```python
from build123d import *

# Parameters (mm, degrees)
SKETCH1_W              = 25.4
SKETCH1_H              = 25.4
SKETCH1_W_2            = 19.05
SKETCH1_H_2            = 19.05
BOSS_EXTRUDE1_DEPTH    = 347.345
F_10_CLEARANCE_HOLE1_D = 5.1054
F_10_CLEARANCE_HOLE2_D = 5.1054


with BuildPart() as part:
    # Sketch1 → Boss-Extrude1 (new body)
    with BuildSketch(Plane(origin=(0, 0, 0), x_dir=(1, 0, 0), z_dir=(0, 1, 0))):
        Rectangle(SKETCH1_W, SKETCH1_H)
        Rectangle(SKETCH1_W_2, SKETCH1_H_2, mode=Mode.SUBTRACT)
    extrude(amount=BOSS_EXTRUDE1_DEPTH)

    # #10 Clearance Hole1 (through all)
    with Locations(Plane.XY.offset(12.7)):
        with Locations((0, 283.845), (0, 12.7), (0, 38.1), (0, 63.5), (0, 334.645), (0, 309.245)):
            Hole(F_10_CLEARANCE_HOLE1_D / 2)

    # #10 Clearance Hole2 (through all)
    with Locations(Plane(origin=(-1665.705302189, -475.547296868, 15.875), x_dir=(1, 0, 0), z_dir=(0, 0, 1))):
        with Locations((1665.705300516, 564.447296868), (1665.705300516, 733.992296868)):
            Hole(F_10_CLEARANCE_HOLE2_D / 2)


solid = part.part
```
Check sheet for the modelled part. Datum: model origin and axes. Units: mm. A direction names the side the tool comes from. Coordinates: 2 decimals unless noted, no trailing zeros. Loops run counter-clockwise (first coordinate to the right, second up) from the corner with the lowest first, then second, coordinate; pieces in that order, holes last.
1) Access from +Z, -Z, +X, -X, +Y, -Y to the whole of each face (thin tool, end or side, straight path). Record for faces 1 (the face through (0, 171, 9.525)), 2 (the face through (0, 171, 12.7)).
2) Release check for a two-part mould opening along X. For faces 3 (the face through (-12.7, 171, 0)), 4 (the face through (9.525, 171, 0)), 5 (the face through (0, 171, -12.7)), 6 (the face through (12.7, 171, 0)) record: released by +X, released by -X, zero draft, split by the parting line, or undercut.
3) Sectioned sample at B-B (x = -6.25). Record the boundary of the cut face in (y, z) (3 decimals), and give its area (3 significant figures).
4) Material ranges on probe 1 along X at (y, z) = (88.9, -11.75); probe 2 along X at (y, z) = (258.5, -0.75) (3 decimals), recorded low to high.
5) Sectioned sample at A-A (z = -0.5). Record the boundary of the cut face in (x, y) (3 decimals), and give its area (3 significant figures).
6) Gauge pin test, flat end, axial feed: pin 1 (4 mm diameter, centred on x = 0, y = 258.45, fed in from -Z). Record the tip position at first contact, or that the pin passes through.
7) Sectioned sample at C-C (y = 50). Record the boundary of the cut face in (x, z) (3 decimals), and give its area (3 significant figures).
Check sheet entries:
1. face 1: +Y, -Y
1. face 2: +Z, +X, -X, +Y, -Y
2. face 3: released by -X
2. face 4: undercut
2. face 5: zero draft
2. face 6: released by +X
3. outline: (0, -12.7) - (347.345, -12.7) - (347.345, -9.525) - (0, -9.525) - close; (0, 9.525) - (347.345, 9.525) - (347.345, 12.7) - (0, 12.7) - close
3. area: 2,210 mm2
4. probe 1: x = -12.7 to -2.55, 2.55 to 12.7
4. probe 2: x = -12.7 to -9.525, 9.525 to 12.7
5. outline: (-12.7, 0) - (-9.525, 0) - (-9.525, 347.345) - (-12.7, 347.345) - close; (9.525, 0) - (12.7, 0) - (12.7, 347.345) - (9.525, 347.345) - close
5. area: 2,210 mm2
6. pin 1: passes through
7. outline: (-12.7, -12.7) - (12.7, -12.7) - (12.7, 12.7) - (-12.7, 12.7) - close; hole (-9.525, -9.525) - (9.525, -9.525) - (9.525, 9.525) - (-9.525, 9.525) - close
7. area: 282 mm2
